Check sheet for the drawn part. Datum: minimum x, y, z corner. Units: mm. A direction names the side the tool comes from. Round coordinates to 2 decimals unless told otherwise and drop trailing zeros. Write each loop counter-clockwise with the first axis right and the second up, starting at its lowest first coordinate (ties: lowest second). Pieces come first, ordered by that corner, then holes. Notation, with made-up numbers: M 43,-1.5 L 98,-1.5 A25 cw 98,28.5 Z; hole C 31,28.5 d4. An arc over 180 degrees is marked long. Answer in a Markdown table with one row per item. Add a question column.
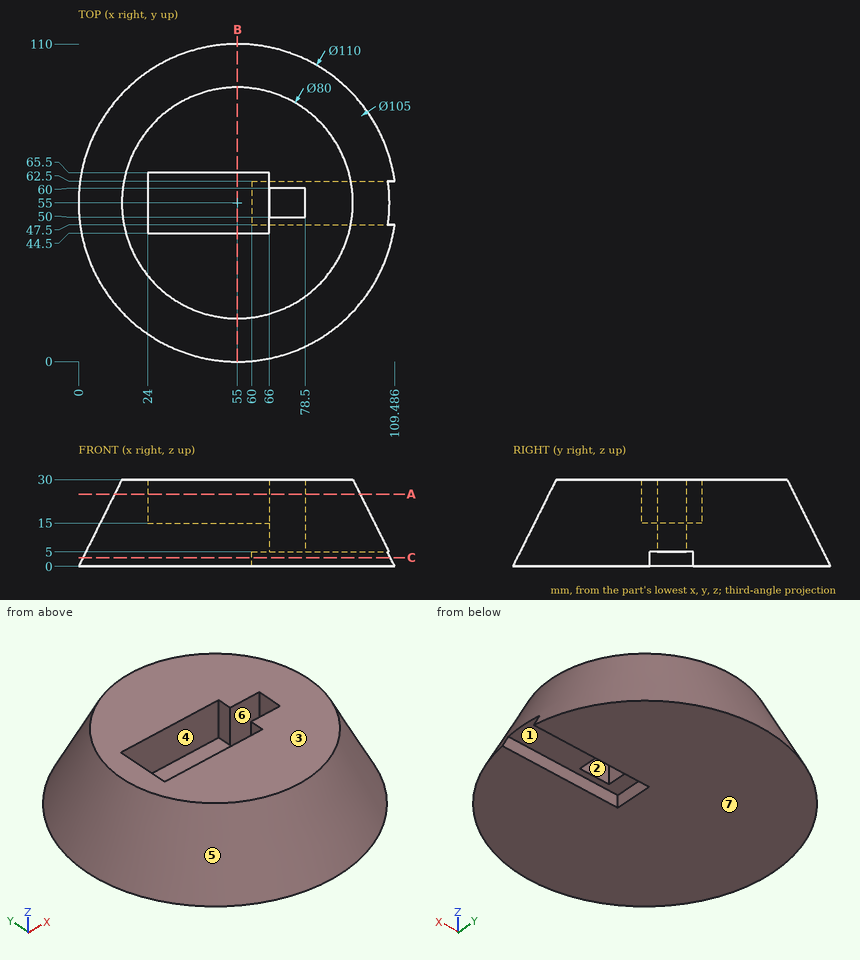
Item 1: Section check B-B, the plane x = 55. Record the boundary of the cut face in (y, z).
Item 2: Access from +Z, -Z, +X, -X, +Y, -Y to the whole of each face (thin tool, end or side, straight path). Record for the marked faces 1, 2, 3 and 4.
Item 3: Gauge pin test, flat ends, axial feed: pin 1 Ø10 at (x, y) = (91, 76.5) entering from +Z; pin 2 Ø11 at (y, z) = (55.5, 16.5) entering from -X; pin 3 Ø4.5 at (y, z) = (64, 21) entering from -X; pin 4 Ø5.5 at (x, z) = (76.5, 1.5) entering from -Y. Record the tip position at first contact, or that the pin passes through.
Item 4: Section check A-A, the plane z = 25. Record the boundary of the cut face in (x, y), and give its area (3 significant figures).
Item 5: Mould release check, pull along Y, two halves, no side actions. Record for the marked faces 5, 6 and 7: +Y half, -Y half, draft (parallel to the pull), parting line (faces both ways), or undercut.
Item 6: Section check C-C, the plane z = 3. Record the boundary of the cut face in (x, y), and give its area (3 significant figures).
Item 7: Scan lines: probe 1 along Y at (x, z) = (76, 19); probe 2 along X at (y, z) = (65, 24); probe 3 along Y at (x, z) = (67, 13). Record each from-to range of solid material in increasing order. Write a range as from..to.
Result sheet:
| question | item | result |
|---|---|---|
| 1 | outline | M 0,0 L 110,0 L 95,30 L 65.5,30 L 65.5,15 L 44.5,15 L 44.5,30 L 15,30 Z |
| 2 | face 1 | -Z, +X |
| 2 | face 2 | +Z, -Z |
| 2 | face 3 | +Z, +X, -X, +Y, -Y |
| 2 | face 4 | +Z |
| 3 | pin 1 | stops at z = 30 |
| 3 | pin 2 | stops at x = 5.5 |
| 3 | pin 3 | stops at x = 10.19 |
| 3 | pin 4 | stops at y = 3.46 |
| 4 | outline | C 55,55 d85; hole M 24,44.5 L 66,44.5 L 66,50 L 78.5,50 L 78.5,60 L 66,60 L 66,65.5 L 24,65.5 Z |
| 4 | area | 4,670 mm^2 |
| 5 | face 5 | parting line |
| 5 | face 6 | undercut |
| 5 | face 7 | draft |
| 6 | outline | M 60,47.5 L 60,62.5 L 107.97,62.5 A53.5 ccw long 107.97,47.5 Z |
| 6 | area | 8,270 mm^2 |
| 7 | probe 1 | y = 14.64..50, 60..95.36 |
| 7 | probe 2 | x = 13.18..24, 66..96.82 |
| 7 | probe 3 | y = 8.01..50, 60..101.99 |
